```python
from build123d import *

# Parameters (mm, degrees)
SKETCH1_W           = 66
SKETCH1_H           = 35.3
SKETCH1_R           = 1.65
BOSS_EXTRUDE1_DEPTH = 4
SKETCH2_R           = 0.85
CUT_EXTRUDE1_DEPTH  = 4
SKETCH3_W           = 24
SKETCH3_H           = 23
CUT_EXTRUDE2_DEPTH  = 3


with BuildPart() as part:
    # Sketch1 → Boss-Extrude1 (new body)
    with BuildSketch(Plane(origin=(0, 0, 0), x_dir=(1, 0, 0), z_dir=(0, 1, 0))):
        with Locations((33, 17.65)):
            Rectangle(SKETCH1_W, SKETCH1_H)
        with Locations(Location((3, 32.15, 0), (0, 0, 270))):
            Circle(SKETCH1_R, mode=Mode.SUBTRACT)
        with Locations(Location((3, 3.15, 0), (0, 0, 270))):
            Circle(SKETCH1_R, mode=Mode.SUBTRACT)
        with Locations(Location((63, 3.15, 0), (0, 0, 270))):
            Circle(SKETCH1_R, mode=Mode.SUBTRACT)
        with Locations(Location((63, 32.15, 0), (0, 0, 270))):
            Circle(SKETCH1_R, mode=Mode.SUBTRACT)
    extrude(amount=BOSS_EXTRUDE1_DEPTH)

    # Sketch2 → Cut-Extrude1 (cut)
    with BuildSketch(Plane(origin=(0, 4, 0), x_dir=(1, 0, 0), z_dir=(0, 1, 0))):
        with Locations(Location((19, 31.15, 0), (0, 0, 270))):
            Circle(SKETCH2_R)
        with Locations(Location((47, 31.15, 0), (0, 0, 270))):
            Circle(SKETCH2_R)
        with Locations(Location((47, 4.15, 0), (0, 0, 270))):
            Circle(SKETCH2_R)
        with Locations(Location((19, 4.15, 0), (0, 0, 270))):
            Circle(SKETCH2_R)
    extrude(amount=-CUT_EXTRUDE1_DEPTH, mode=Mode.SUBTRACT)

    # Sketch3 → Cut-Extrude2 (cut)
    with BuildSketch(Plane(origin=(0, 4, 0), x_dir=(1, 0, 0), z_dir=(0, 1, 0))):
        with Locations((33, 17.65)):
            Rectangle(SKETCH3_W, SKETCH3_H)
    extrude(amount=-CUT_EXTRUDE2_DEPTH, mode=Mode.SUBTRACT)


solid = part.part
```
For this review, take the finished solid that the model builds, in its own axes (mm). A direction names the side the tool comes from. Give positions to 0.01 mm unless a question says otherwise; leave off trailing zeros. Write each loop counter-clockwise with the first axis right and the second up, starting at its lowest first coordinate (ties: lowest second). Pieces come first, ordered by that corner, then holes. Notation, with made-up numbers: M 33.5,-9 L 40.5,-9 A32 ccw 40.5,19 Z; hole C 50,23 d2. An arc over 180 degrees is marked long. Answer as a JSON object with one key per item and string values. Group by question number.
Item 1: Draft analysis for pull direction Z (two halves, no side actions). For faces 3 (the flat face through (33, 3, -29.15)), 4 (the flat face through (33, 2, 0)), 5 (the flat face through (66, 2, -17)), state which applies: +Z half, -Z half, draft (parallel to the pull), parting line (faces both ways), or undercut.
Item 2: For probe 1 along X at (y, z) = (2.3, -3.15); probe 2 along X at (y, z) = (1.8, -27.5); probe 3 along X at (y, z) = (2.8, -31.5), list the stretches that pass through material, from the lowest coordinate up. Write a range as [from, to].
Item 3: Consider section A-A on x = 3. Write out the cut boundary in (y, z), plus the area to 3 significant figures.
Item 4: Consider section C-C on z = -7. Write out the cut boundary in (x, y), plus the area to 3 significant figures.
Item 5: Consider section B-B on y = 2.2. Count the separate pieces of the cut face and the enclosed holes in it, plus the area to 3 significant figures.
Item 6: Tool access review of faces 1 (the flat face through (45, 3, -17)), 2 (the cylindrical face through (61.39, 1.97, -3.51)): name each direction out of +Z, -Z, +X, -X, +Y, -Y from which nothing blocks a thin tool from reaching the whole face with its end or side.
Item 7: Consider section D-D on z = -31.15. Write out the cut boundary in (x, y).
Check result:
{
 "1": {"face 3": "undercut", "face 4": "+Z half", "face 5": "draft"},
 "2": {"probe 1": "x = [0, 1.35], [4.65, 61.35], [64.65, 66]", "probe 2": "x = [0, 21], [45, 66]", "probe 3": "x = [0, 1.48], [4.52, 18.23], [19.77, 46.23], [47.77, 61.48], [64.52, 66]"},
 "3": {"outline": "M 0,-35.3 L 4,-35.3 L 4,-33.8 L 0,-33.8 Z; M 0,-30.5 L 4,-30.5 L 4,-4.8 L 0,-4.8 Z; M 0,-1.5 L 4,-1.5 L 4,0 L 0,0 Z", "area": "115 mm^2"},
 "4": {"outline": "M 0,0 L 66,0 L 66,4 L 45,4 L 45,1 L 21,1 L 21,4 L 0,4 Z", "area": "192 mm^2"},
 "5": {"separate pieces": "1", "enclosed holes": "9", "area": "1,730 mm^2"},
 "6": {"face 1": "+Y", "face 2": "+Y, -Y"},
 "7": {"outline": "M 0,0 L 1.69,0 L 1.69,4 L 0,4 Z; M 4.31,0 L 18.15,0 L 18.15,4 L 4.31,4 Z; M 19.85,0 L 46.15,0 L 46.15,4 L 19.85,4 Z; M 47.85,0 L 61.69,0 L 61.69,4 L 47.85,4 Z; M 64.31,0 L 66,0 L 66,4 L 64.31,4 Z"}
}
